Design review of the part built by this model. Coordinates are the model's own, in mm. Face numbers are marked on the shaded views. A direction names the side the tool comes from. Give positions to 0.01 mm unless a question says otherwise; leave off trailing zeros. Loops run counter-clockwise (first coordinate to the right, second up) from the corner with the lowest first, then second, coordinate; pieces in that order, holes last. Notation, with made-up numbers: (43, -13.75) - (56, -13.75) arc R10 ccw to (56, -8.75) - close; hole circle Ø10 at (-27, 83.5). An arc over 180 degrees is marked (long way). Write each question's results on one line, items separated by ' | '.
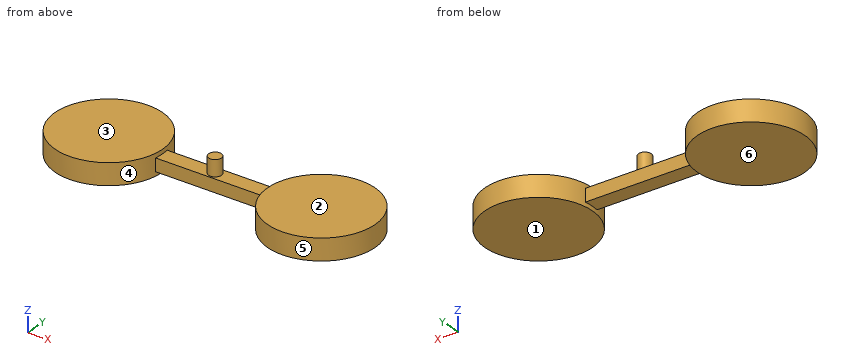
```python
from build123d import *

# Parameters (mm, degrees)
CYLINDER142_R     = 2.5
CYLINDER142_DEPTH = 1
CYLINDER141_R     = 2.5
CYLINDER141_DEPTH = 1
CYLINDER140_R     = 0.3
CYLINDER140_DEPTH = 0.75
BOX_W             = 10
BOX_H             = 0.75
BOX_DEPTH         = 0.6


with BuildPart() as obj1:
    # Cylinder142 → Cylinder142 (new body)
    with BuildSketch(Plane(origin=(5, 0, -0.5), x_dir=(1, 0, 0), z_dir=(0, 0, 1))):
        Circle(CYLINDER142_R)
    extrude(amount=CYLINDER142_DEPTH)


with BuildPart() as obj2:
    # Cylinder141 → Cylinder141 (new body)
    with BuildSketch(Plane(origin=(-5, 0, -0.5), x_dir=(1, 0, 0), z_dir=(0, 0, 1))):
        Circle(CYLINDER141_R)
    extrude(amount=CYLINDER141_DEPTH)


with BuildPart() as nozzle_od:
    # Cylinder140 → Cylinder140 (new body)
    with BuildSketch(Plane.XY.offset(0.3)):
        Circle(CYLINDER140_R)
    extrude(amount=CYLINDER140_DEPTH)


with BuildPart() as fusion:
    # Box → Box (new body)
    with BuildSketch(Plane(origin=(-5, -0.375, -0.3), x_dir=(1, 0, 0), z_dir=(0, 0, 1))):
        with Locations((5, 0.375)):
            Rectangle(BOX_W, BOX_H)
    extrude(amount=BOX_DEPTH)

    # Fusion: union obj1, obj2, Nozzle_OD
    add(obj1.part)
    add(obj2.part)
    add(nozzle_od.part)


solid = fusion.part
```
Item 1: Wall thickness on probe 1 along Z at (x, y) = (6, 1.8); probe 2 along X at (y, z) = (1.5, 0.2); probe 3 along X at (y, z) = (-1.7, -0.1): over which ranges is each line inside the solid? List them lowest first.
Output values:
probe 1: z = -0.5 to 0.5 | probe 2: x = -7 to -3, 3 to 7 | probe 3: x = -6.83 to -3.17, 3.17 to 6.83
Item 2: Draft analysis for pull direction X (two halves, no side actions). For the marked faces 4, 5 and 6, state which applies: +X half, -X half, draft (parallel to the pull), parting line (faces both ways), or undercut.
Output values:
face 4: undercut | face 5: undercut | face 6: draft
Item 3: Tool access review of the marked faces 1, 2 and 3: name each direction out of +Z, -Z, +X, -X, +Y, -Y from which nothing blocks a thin tool from reaching the whole face with its end or side.
Output values:
face 1: -Z, +X, -X, +Y, -Y | face 2: +Z, +X, +Y, -Y | face 3: +Z, -X, +Y, -Y
Item 4: Clearance check with a flat-ended pin moving along its axis: P1, Ø1, axis at x = 0.5, y = 1, coming from the +Z side. State where the tip first meets the part, or that it passes through.
Output values:
P1: passes through
Item 5: We need section C-C on x = 0. Give the boundary of the cut face in (y, z) (3 decimals).
Output values:
outline: (-0.375, -0.3) - (0.375, -0.3) - (0.375, 0.3) - (0.3, 0.3) - (0.3, 1.05) - (-0.3, 1.05) - (-0.3, 0.3) - (-0.375, 0.3) - close
Item 6: We need section B-B on y = 2.15. Give the boundary of the cut face in (x, z).
Output values:
outline: (-6.28, -0.5) - (-3.72, -0.5) - (-3.72, 0.5) - (-6.28, 0.5) - close; (3.72, -0.5) - (6.28, -0.5) - (6.28, 0.5) - (3.72, 0.5) - close
Item 7: We need section A-A on y = 0. Give the boundary of the cut face in (x, z).
Output values:
outline: (-7.5, -0.5) - (-2.5, -0.5) - (-2.5, -0.3) - (2.5, -0.3) - (2.5, -0.5) - (7.5, -0.5) - (7.5, 0.5) - (2.5, 0.5) - (2.5, 0.3) - (0.3, 0.3) - (0.3, 1.05) - (-0.3, 1.05) - (-0.3, 0.3) - (-2.5, 0.3) - (-2.5, 0.5) - (-7.5, 0.5) - close
Item 8: We need section D-D on z = 0.7. Give the boundary of the cut face in (x, y), then the cut area to 3 significant figures.
Output values:
outline: circle Ø0.6 at (0, 0) | area: 0.283 mm²
